```python
from build123d import *

# Parameters (mm, degrees)
SKETCH_1_R          = 9.5
EXTRUDE_1_DEPTH     = 37
SKETCH_2_R          = 7.5
CUT_EXTRUDE_1_DEPTH = 7
CHAMFER_1_SIZE      = 1
CHAMFER_2_SIZE      = 0.5


with BuildPart() as part:
    # 草图1 → 凸台-拉伸1 (new body)
    with BuildSketch(Plane(origin=(0, 0, 0), x_dir=(1, 0, 0), z_dir=(0, 1, 0))):
        with Locations(Location((0, 0, 0), (0, 0, 270))):
            Circle(SKETCH_1_R)
    extrude(amount=EXTRUDE_1_DEPTH)

    # 草图2 → 切除-拉伸1 (cut)
    with BuildSketch(Plane.XZ):
        with Locations(Location((0, 0, 0), (0, 0, 270))):
            Circle(SKETCH_2_R)
    extrude(amount=-CUT_EXTRUDE_1_DEPTH, mode=Mode.SUBTRACT)

    # 倒角1
    chamfer_1_edges = [part.edges().sort_by_distance(p)[0] for p in [
        (0, 37, -9.5),
    ]]
    chamfer(chamfer_1_edges, length=CHAMFER_1_SIZE)

    # 倒角2
    chamfer_2_edges = [part.edges().sort_by_distance(p)[0] for p in [
        (0, 0, 7.5),
    ]]
    chamfer(chamfer_2_edges, length=CHAMFER_2_SIZE)


solid = part.part
```
Can you work these out from the model? Positions are in its coordinate system, mm. A direction names the side the tool comes from. Round coordinates to 2 decimals unless told otherwise and drop trailing zeros. Loops run counter-clockwise (first coordinate to the right, second up) from the corner with the lowest first, then second, coordinate; pieces in that order, holes last. Notation, with made-up numbers: (84, -3.5) -> (138, -3.5) arc R29 cw to (138, 32.5) -> close; hole circle Ø7 at (88.25, 73.25). An arc over 180 degrees is marked (long way). One line per item, written item: value. Start each with the question number.
1. If we section it at C-C, the plane y = 6: Write out the boundary of the cut face in (x, z).
2. If we section it at A-A, the plane x = 0: Write out the boundary of the cut face in (y, z).
3. If I drill on probe 1 along X at (y, z) = (4, 0); probe 2 along Y at (x, z) = (-0.5, -5.75); probe 3 along Z at (x, y) = (0.25, 30.5), over which ranges is the centre line in solid material (lowest first)?
4. For faces 1 (the flat face through (0, 37, 0)), 2 (the flat face through (0, 7, 0)), which set-ups out of +Z, -Z, +X, -X, +Y, -Y let a thin tool reach every point of the face, with its end or its side?
5. If we mould it in two halves opening along X, with no side actions, what happens to faces 3 (the cylindrical face through (-5.78, 17.75, -7.54)), 4 (the cylindrical face through (0.33, 3.704, 7.493)), 5 (the flat face through (-7, 0, -4.3))? For each: pulls with the +X half, pulls with the -X half, needs draft (parallel to the pull), parting line crosses it, or undercut.
6. If we section it at B-B, the plane z = 0: Write out the boundary of the cut face in (x, y), then the cut area to 3 significant figures.
7. For pin 1 (5 mm diameter, centred on y = 19, z = -3, fed in from +X); pin 2 (4 mm diameter, centred on y = 12.5, z = -7, fed in from -X); pin 3 (3 mm diameter, centred on x = -0.5, z = -2, fed in from -Y), each with a flat end and sliding along its axis, tell me the tip position at first contact or that it passes through.
Calculated:
1. outline: circle Ø19 at (0, 0); hole circle Ø15 at (0, 0)
2. outline: (0, -9.5) -> (36, -9.5) -> (37, -8.5) -> (37, 8.5) -> (36, 9.5) -> (0, 9.5) -> (0, 8) -> (0.5, 7.5) -> (7, 7.5) -> (7, -7.5) -> (0.5, -7.5) -> (0, -8) -> close
3. probe 1: x = -9.5 to -7.5, 7.5 to 9.5
3. probe 2: y = 7 to 37
3. probe 3: z = -9.5 to 9.5
4. face 1: +Z, -Z, +X, -X, +Y
4. face 2: -Y
5. face 3: parting line crosses it
5. face 4: undercut
5. face 5: needs draft
6. outline: (-9.5, 0) -> (-8, 0) -> (-7.5, 0.5) -> (-7.5, 7) -> (7.5, 7) -> (7.5, 0.5) -> (8, 0) -> (9.5, 0) -> (9.5, 36) -> (8.5, 37) -> (-8.5, 37) -> (-9.5, 36) -> close
6. area: 597 mm²
7. pin 1: stops at x = 9.49
7. pin 2: stops at x = -8.08
7. pin 3: stops at y = 7
